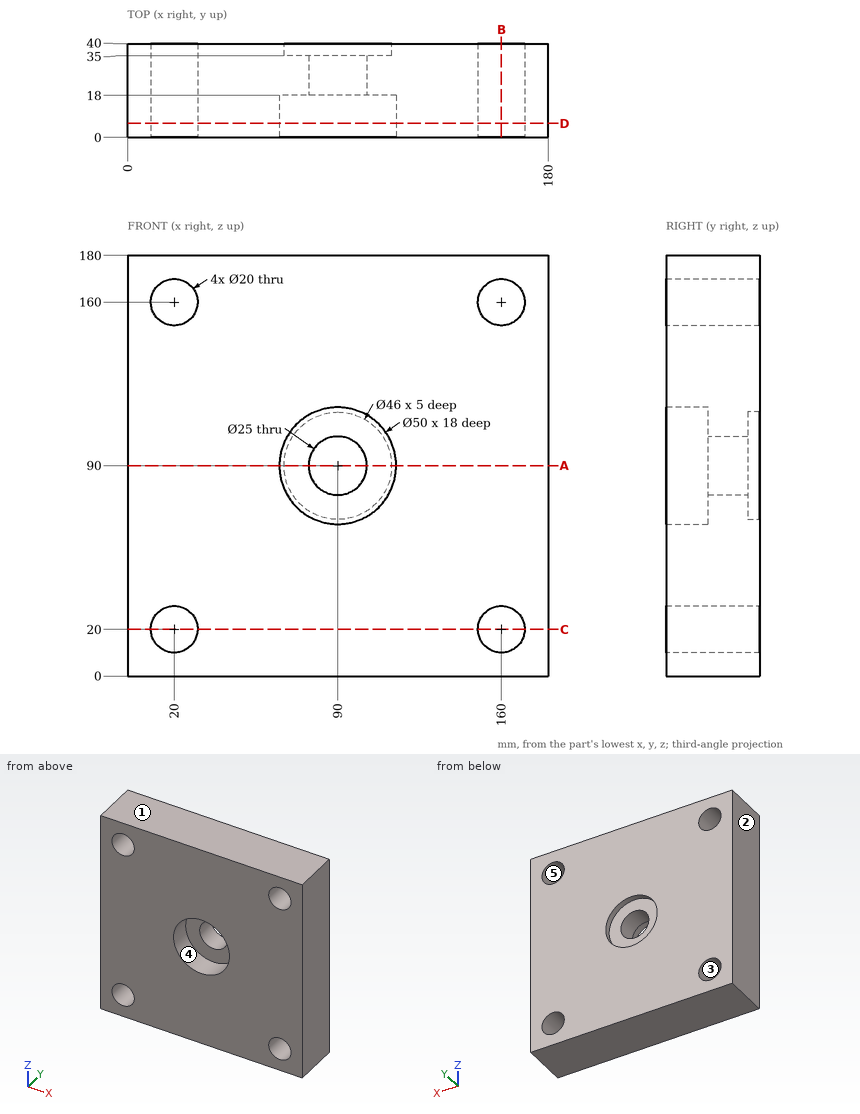
Study the drawing (mm; zero at the part's minimum x, y, z) and answer. A direction names the side the tool comes from. Coordinates: 2 decimals unless noted, no trailing zeros. Loops run counter-clockwise (first coordinate to the right, second up) from the corner with the lowest first, then second, coordinate; pieces in that order, holes last. Notation, with made-up numbers: (3, 9) -> (9, 9) arc R35 ccw to (9, 42) -> close; hole circle Ø4 at (64, 25.25). An arc over 180 degrees is marked (long way). Write item = value, one per line. Start each with the question number.
1) The part is cut by section B-B, the plane x = 160. Determine the outline of the cut face in (y, z), plus the area to 3 significant figures.
2) The mould has two halves that part along X. Classify the marked faces 1, 2 and 3: pulls with the +X half, pulls with the -X half, needs draft (parallel to the pull), parting line crosses it, or undercut.
3) For the marked faces 4 and 5, determine the directions among +Z, -Z, +X, -X, +Y, -Y from which every point of the face is accessible in a straight line to the end or side of a thin tool.
4) The part is cut by section C-C, the plane z = 20. Determine the outline of the cut face in (x, y).
5) Find the intervals of material crossed by L1, parallel to X at y = 22, z = 20; L2, parallel to Z at x = 164.5, y = 19; L3, parallel to X at y = 5, z = 90, in increasing order. Write a range as from..to.
6) The part is cut by section A-A, the plane z = 90. Determine the outline of the cut face in (x, y).
7) The part is cut by section D-D, the plane y = 6. Determine the outline of the cut face in (x, z), plus the area to 3 significant figures.
8) Given P1, Ø5, axis at y = 24, z = 78, coming from the -X side; P2, Ø15, axis at x = 80, z = 102, coming from the -Y side, each flat-ended and moving along its own axis, determine where each tip first touches the part or whether it passes through.
Result:
q1.outline = (0, 0) -> (40, 0) -> (40, 10) -> (0, 10) -> close; (0, 30) -> (40, 30) -> (40, 150) -> (0, 150) -> close; (0, 170) -> (40, 170) -> (40, 180) -> (0, 180) -> close
q1.area = 5,600 mm²
q2.face_1 = needs draft
q2.face_2 = pulls with the -X half
q2.face_3 = undercut
q3.face_4 = -Y
q3.face_5 = +Y, -Y
q4.outline = (0, 0) -> (10, 0) -> (10, 40) -> (0, 40) -> close; (30, 0) -> (150, 0) -> (150, 40) -> (30, 40) -> close; (170, 0) -> (180, 0) -> (180, 40) -> (170, 40) -> close
q5.L1 = 0..10, 30..150, 170..180
q5.L2 = 0..11.07, 28.93..151.07, 168.93..180
q5.L3 = 0..65, 115..180
q6.outline = (0, 0) -> (65, 0) -> (65, 18) -> (77.5, 18) -> (77.5, 35) -> (67, 35) -> (67, 40) -> (0, 40) -> close; (102.5, 18) -> (115, 18) -> (115, 0) -> (180, 0) -> (180, 40) -> (113, 40) -> (113, 35) -> (102.5, 35) -> close
q7.outline = (0, 0) -> (180, 0) -> (180, 180) -> (0, 180) -> close; hole circle Ø20 at (20, 20); hole circle Ø20 at (20, 160); hole circle Ø50 at (90, 90); hole circle Ø20 at (160, 20); hole circle Ø20 at (160, 160)
q7.area = 29,200 mm²
q8.P1 = 0
q8.P2 = 18
